Study the drawing (mm; zero at the part's minimum x, y, z) and answer. A direction names the side the tool comes from. Round coordinates to 2 decimals unless told otherwise and drop trailing zeros. Loops run counter-clockwise (first coordinate to the right, second up) from the corner with the lowest first, then second, coordinate; pieces in that order, holes last. Notation, with made-up numbers: (-16.5, -35) - (-5.5, -35) arc R20 cw to (-5.5, -14) - close; hole circle Ø9 at (-17, -3). An arc over 180 degrees is marked (long way). Use CSV: the item, a comma, the result in double quotes. Start each with the question number.
1. Consider line 1 along X through (y, z) = (3, 7.75); line 2 along X through (y, z) = (9.5, 1). Determine where each line is inside the solid, lowest interval first.
2. Determine the mould class of the marked faces 4, 5 and 6 for opening direction Y: +Y half, -Y half, draft (parallel to the pull), parting line (faces both ways), or undercut.
3. Find section A-A (z = 2.25). Give the vertices of the cut face in (x, y) (3 decimals), and give its area (3 significant figures).
4. Find section D-D (y = 8). Give the vertices of the cut face in (x, z) (3 decimals), and give its area (3 significant figures).
5. Find section B-B (y = 12). Give the vertices of the cut face in (x, z) (3 decimals), and give its area (3 significant figures).
6. A tool of negligible diameter and unlimited length cuts with its end or side. For the marked faces 1, 2 and 3, from which of +Z, -Z, +X, -X, +Y, -Y can it reach the whole face along a straight path? Write none if from no direction.
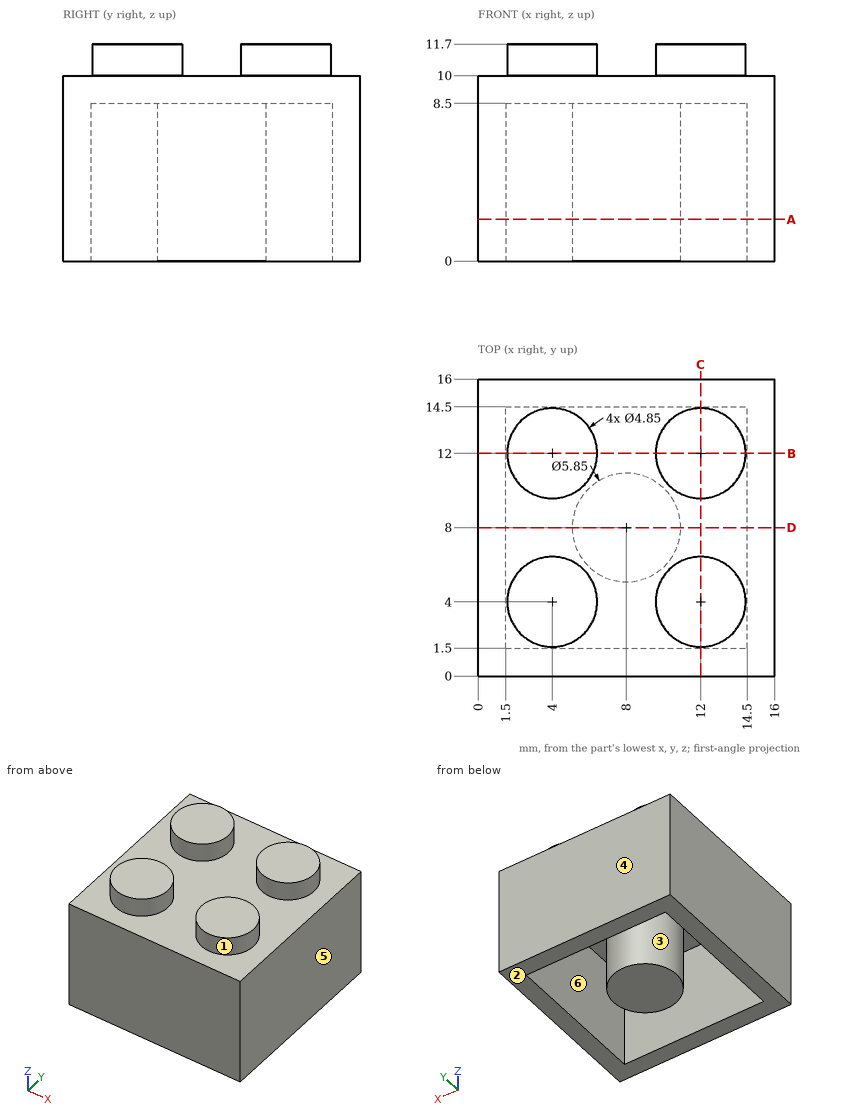
Filled sheet:
1,line 1,"x = 0 to 1.5, 14.5 to 16"
1,line 2,"x = 0 to 1.5, 5.49 to 10.51, 14.5 to 16"
2,face 4,"+Y half"
2,face 5,"draft"
2,face 6,"undercut"
3,outline,"(0, 0) - (16, 0) - (16, 16) - (0, 16) - close; circle Ø5.85 at (8, 8); hole (1.5, 1.5) - (14.5, 1.5) - (14.5, 14.5) - (1.5, 14.5) - close"
3,area,"114 mm²"
4,outline,"(0, 0) - (1.5, 0) - (1.5, 8.5) - (5.075, 8.5) - (5.075, 0) - (10.925, 0) - (10.925, 8.5) - (14.5, 8.5) - (14.5, 0) - (16, 0) - (16, 10) - (0, 10) - close"
4,area,"99.2 mm²"
5,outline,"(0, 0) - (1.5, 0) - (1.5, 8.5) - (14.5, 8.5) - (14.5, 0) - (16, 0) - (16, 10) - (14.425, 10) - (14.425, 11.7) - (9.575, 11.7) - (9.575, 10) - (6.425, 10) - (6.425, 11.7) - (1.575, 11.7) - (1.575, 10) - (0, 10) - close"
5,area,"66.0 mm²"
6,face 1,"+Z"
6,face 2,"-Z, +X, -X, +Y, -Y"
6,face 3,"-Z"
